For this review, take the finished solid that the model builds, in its own axes (mm). Coordinates: 2 decimals unless noted, no trailing zeros. Order: outer loops, then holes, each group sorted by start corner. A loop starts at its lowest first (then second) coordinate and runs counter-clockwise, first axis right, second up. Notation, with made-up numbers: (-33.75, 41) -> (18.25, 41) arc R4 ccw to (18.25, 47) -> close; hole circle Ø2 at (80, -9.5). An arc over 180 degrees is marked (long way). Write item = value, one per line. Start each with the question number.
1) Consider section A-A on z = -549.5. Give the boundary of the cut face in (x, y), and give its area (3 significant figures).
2) Consider section B-B on y = 21. Give the boundary of the cut face in (x, z), and give its area (3 significant figures).
3) Wall thickness on probe 1 along X at (y, z) = (22.75, -572.5); probe 2 along Z at (x, y) = (447.5, 18); probe 3 along Z at (x, y) = (486, 22.75): over which ranges is each line inside the solid? List them lowest first. Write a range as [from, to].
from build123d import *

# Parameters (mm, degrees)
SKETCH_1_W          = 794
SKETCH_1_H          = 8
EXTRUDE_1_DEPTH     = 600
CUT_EXTRUDE_1_DEPTH = 1018.353969246


with BuildPart() as part:
    # 草图1 → 凸台-拉伸1 (new body)
    with BuildSketch(Plane.XY):
        with Locations((424.550423736, 20)):
            Rectangle(SKETCH_1_W, SKETCH_1_H)
    extrude(amount=-EXTRUDE_1_DEPTH)

    # 草图2 → 切除-拉伸1 (cut, through all)
    with BuildSketch(Plane.XZ.offset(-16)):
        with BuildLine():
            Line((396, -443), (484, -443))
            ThreePointArc((484, -443), (487.535533906, -444.464466094), (489, -448))
            Line((489, -448), (489, -603))
            Line((489, -603), (391, -603))
            Line((391, -603), (391, -448))
            ThreePointArc((391, -448), (392.464466094, -444.464466094), (396, -443))
        make_face()
    extrude(amount=-CUT_EXTRUDE_1_DEPTH, mode=Mode.SUBTRACT)


solid = part.part
Answer sheet:
q1.outline = (27.55, 16) -> (391, 16) -> (391, 24) -> (27.55, 24) -> close; (489, 16) -> (821.55, 16) -> (821.55, 24) -> (489, 24) -> close
q1.area = 5,570 mm2
q2.outline = (27.55, -600) -> (391, -600) -> (391, -448) arc R5 cw to (396, -443) -> (484, -443) arc R5 cw to (489, -448) -> (489, -600) -> (821.55, -600) -> (821.55, 0) -> (27.55, 0) -> close
q2.area = 461,000 mm2
q3.probe_1 = [27.55, 391], [489, 821.55]
q3.probe_2 = [-443, 0]
q3.probe_3 = [-443.42, 0]
